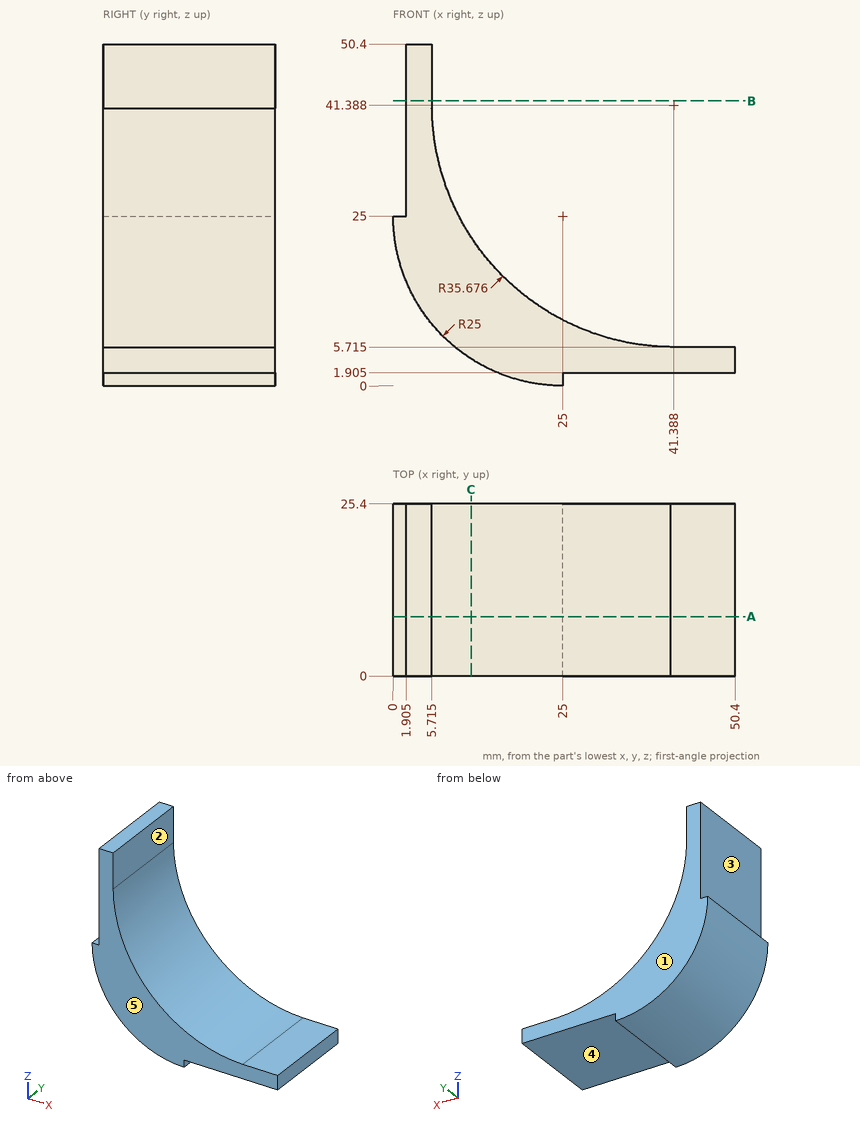
For this review, use the dimensioned drawing (mm, ordinates from the lowest corner) and the shaded views. A direction names the side the tool comes from. Give positions to 0.01 mm unless a question says otherwise; leave off trailing zeros. Loops run counter-clockwise (first coordinate to the right, second up) from the corner with the lowest first, then second, coordinate; pieces in that order, holes last. Notation, with made-up numbers: (7.5, 56) -> (19.5, 56) arc R19 cw to (19.5, 76) -> close; hole circle Ø3 at (70.25, 41.25). An arc over 180 degrees is marked (long way). Use CSV: the item, a comma, the result in double quotes.
1. Consider section C-C, the plane x = 11.5. Write out the cut boundary in (y, z), then the cut area to 3 significant figures.
Result:
outline,"(0, 3.96) -> (25.4, 3.96) -> (25.4, 21.91) -> (0, 21.91) -> close"
area,"456 mm²"
2. To check wall thickness, follow probe 1 along Z at (x, y) = (43, 10) (1 decimal); probe 2 along X at (y, z) = (16.75, 21.5) (1 decimal); probe 3 along Z at (x, y) = (34, 17) (1 decimal). State the ranges of each line that lie inside material, in increasing order. Write a range as from..to.
Result:
probe 1,"z = 1.9..5.7"
probe 2,"x = 0.2..11.8"
probe 3,"z = 1.9..6.5"
3. Machinability: for the marked faces 1, 2, 3, 4 and 5, which of the approach directions +Z, -Z, +X, -X, +Y, -Y give a long, thin tool a straight path to every point of the face, cutting with its end or side? Answer none if there is none.
Result:
face 1,"+Z, -Z, +X, -X, +Y"
face 2,"+Z, +X, +Y, -Y"
face 3,"+Z, -X, +Y, -Y"
face 4,"-Z, +X, +Y, -Y"
face 5,"+Z, -Z, +X, -X, -Y"
4. Consider section B-B, the plane z = 42. Write out the cut boundary in (x, y) (1 decimal).
Result:
outline,"(1.9, 0) -> (5.7, 0) -> (5.7, 25.4) -> (1.9, 25.4) -> close"
5. Consider section A-A, the plane y = 8.75. Write out the cut boundary in (x, z) (1 decimal).
Result:
outline,"(0, 25) arc R25 ccw to (25, 0) -> (25, 1.9) -> (50.4, 1.9) -> (50.4, 5.7) -> (40.9, 5.7) arc R35.7 cw to (5.7, 40.9) -> (5.7, 50.4) -> (1.9, 50.4) -> (1.9, 25) -> close"
6. For P1, Ø0.6, axis at y = 14.5, z = 0.5, coming from the +X side; P2, Ø12, axis at y = 15, z = 22, coming from the +X side (1 decimal); P3, Ø1.5, axis at x = 1, y = 14.5, coming from the +Z side, all flat-tipped, find the tip position at first contact; note any pin that passes through.
Result:
P1,"stops at x = 25"
P2,"stops at x = 16.3"
P3,"stops at z = 25"
